```python
from build123d import *

# Parameters (mm, degrees)
SKETCH_2_R                   = 22.5
EXTRUDE_2_DEPTH              = 2
SKETCH_22_R                  = 10
CUT_EXTRUDE_1_DEPTH          = 2
FILLET_4_R                   = 0.2
SKETCH_54_R                  = 22.5
EXTRUDE_6_DEPTH              = 11
SKETCH_55_R                  = 18.5
CUT_EXTRUDE_2_DEPTH          = 8
HOLE_WIZARD_M4_1_D           = 4.5
HOLE_WIZARD_M4_1_CBORE_D     = 8
HOLE_WIZARD_M4_1_CBORE_DEPTH = 1
PATTERN_CIRCULAR_1_COUNT     = 3
SKETCH_59_R                  = 18.5
SKETCH_59_R_2                = 17.5
EXTRUDE_7_DEPTH              = 1
EXTRUDE_8_DEPTH              = 9
FILLET_6_R                   = 0.3
SKETCH_68_R                  = 9.5
CUT_EXTRUDE_7_DEPTH          = 7
SKETCH_69_R                  = 8.5
CUT_EXTRUDE_8_DEPTH          = 3
FILLET_7_R                   = 0.3


with BuildPart() as part:
    # 스케치2 → 보스-돌출2 (new body)
    with BuildSketch(Plane(origin=(0, 6, 0), x_dir=(1, 0, 0), z_dir=(0, 0, -1))):
        with Locations((0, 6)):
            Circle(SKETCH_2_R)
    extrude(amount=EXTRUDE_2_DEPTH)

    # 스케치22 → 컷-돌출1 (cut)
    with BuildSketch(Plane.XY):
        Circle(SKETCH_22_R)
    extrude(amount=-CUT_EXTRUDE_1_DEPTH, mode=Mode.SUBTRACT)

    # 필렛4
    fillet_4_edges = [part.edges().sort_by_distance(p)[0] for p in [
        (-10, 0, 0),
    ]]
    fillet(fillet_4_edges, radius=FILLET_4_R)

    # 스케치54 → 보스-돌출6 (add)
    with BuildSketch(Plane(origin=(0, 0, -2), x_dir=(-1, 0, 0), z_dir=(0, 0, -1))):
        Circle(SKETCH_54_R)
    extrude(amount=EXTRUDE_6_DEPTH)

    # 스케치55 → 컷-돌출2 (cut)
    with BuildSketch(Plane(origin=(0, 0, -13), x_dir=(-1, 0, 0), z_dir=(0, 0, -1))):
        Circle(SKETCH_55_R)
    extrude(amount=-CUT_EXTRUDE_2_DEPTH, mode=Mode.SUBTRACT)

    # M4 육각 소켓 머리 캡 나사용 카운터보어1 (through all)
    with Locations(Plane(origin=(0, 0, -5), x_dir=(-1, 0, 0), z_dir=(0, 0, -1))):
        with Locations((0, 6)):
            hole_wizard_m4_1 = CounterBoreHole(HOLE_WIZARD_M4_1_D / 2, HOLE_WIZARD_M4_1_CBORE_D / 2, HOLE_WIZARD_M4_1_CBORE_DEPTH)

    # 원형 패턴1: M4 육각 소켓 머리 캡 나사용 카운터보어1 ×3 about axis
    pattern_circular_1_axis = Axis((0, 0, 0), (0, 0, 1))
    for i in range(1, PATTERN_CIRCULAR_1_COUNT):
        add(hole_wizard_m4_1.rotate(pattern_circular_1_axis, i * 360 / PATTERN_CIRCULAR_1_COUNT), mode=Mode.SUBTRACT)

    # 스케치59 → 보스-돌출7 (add)
    with BuildSketch(Plane(origin=(0, 0, -5), x_dir=(-1, 0, 0), z_dir=(0, 0, -1))):
        Circle(SKETCH_59_R)
        Circle(SKETCH_59_R_2, mode=Mode.SUBTRACT)
    extrude(amount=EXTRUDE_7_DEPTH)

    # 스케치60 → 보스-돌출8 (add)
    with BuildSketch(Plane(origin=(0, 0, -13), x_dir=(-1, 0, 0), z_dir=(0, 0, -1))):
        with BuildLine():
            Line((-22.323526687, -2.8125), (-14.882351125, -61.875))
            ThreePointArc((-14.882351125, -61.875), (0, -75), (14.882351125, -61.875))
            Line((14.882351125, -61.875), (22.323526687, -2.8125))
            ThreePointArc((22.323526687, -2.8125), (0, -22.5), (-22.323526687, -2.8125))
        make_face()
    extrude(amount=-EXTRUDE_8_DEPTH)

    # 필렛6
    fillet_6_edges = [part.edges().sort_by_distance(p)[0] for p in [
        (18.5, 0, -6),
    ]]
    fillet(fillet_6_edges, radius=FILLET_6_R)

    # 스케치68 → 컷-돌출7 (cut)
    with BuildSketch(Plane.XY.offset(-4)):
        with Locations((0, -60)):
            Circle(SKETCH_68_R)
    extrude(amount=-CUT_EXTRUDE_7_DEPTH, mode=Mode.SUBTRACT)

    # 스케치69 → 컷-돌출8 (cut, through all)
    with BuildSketch(Plane.XY.offset(-11)):
        with Locations((0, -60)):
            Circle(SKETCH_69_R)
    extrude(amount=-CUT_EXTRUDE_8_DEPTH, mode=Mode.SUBTRACT)

    # 필렛7
    fillet_7_edges = [part.edges().sort_by_distance(p)[0] for p in [
        (-9.5, -60, -11),
    ]]
    fillet(fillet_7_edges, radius=FILLET_7_R)


solid = part.part
```
Here's how the part is built. I have some questions about the finished solid (model axes, mm). A direction names the side the tool comes from. Give positions to 0.01 mm unless a question says otherwise; leave off trailing zeros. Write each loop counter-clockwise with the first axis right and the second up, starting at its lowest first coordinate (ties: lowest second). Pieces come first, ordered by that corner, then holes. Notation, with made-up numbers: (74.25, -21.5) -> (92.25, -21.5) arc R18 cw to (92.25, 13.5) -> close; hole circle Ø10 at (13, 2.5). An arc over 180 degrees is marked (long way). Write each question's results on one line, items separated by ' | '.
Item 1: We'd pull the mould along Y, two halves only. Please class faces 1 (the face through (-3.118, -3.862, -2.986)), 2 (the face through (0, -38, -4)), 3 (the face through (-18.55, -32.76, -8.56)): pulls with the +Y half, pulls with the -Y half, needs draft (parallel to the pull), parting line crosses it, or undercut.
Output:
face 1: undercut | face 2: needs draft | face 3: pulls with the -Y half
Item 2: For pin 1 Ø7 at (x, y) = (5.2, -3) entering from -Z; pin 2 Ø2 at (x, y) = (-13.5, -2) entering from -Z; pin 3 Ø1 at (x, z) = (17, -9) entering from +Y, each with a flat end and sliding along its axis, tell me the tip position at first contact or that it passes through.
Output:
pin 1: stops at z = -4 | pin 2: stops at z = -5 | pin 3: stops at y = 15.3
Item 3: On a 3-axis mill with a long thin cutter (end or side, diameter ignored), from which of +Z, -Z, +X, -X, +Y, -Y can I reach the whole of each face in a straight line? I mean faces 4 (the face through (0, 0, -2)), 5 (the face through (18.655, -31.93, -8.563)), 6 (the face through (15, 10, -6)). Say none if no direction works.
Output:
face 4: +Z | face 5: +Z, -Z, +X, -Y | face 6: -Z
Item 4: Suppose I cut it at C-C on x = 0. Give the number of separate pieces and of enclosed holes in the cut face, plus the area to 3 significant figures.
Output:
separate pieces: 3 | enclosed holes: 0 | area: 540 mm^2
Item 5: If I drill on L1, parallel to Y at x = -2, z = -10; L2, parallel to Y at x = 0, z = -1.3; L3, parallel to Y at x = 7, z = -10.25, over which ranges is the centre line in solid material (lowest first)?
Output:
L1: y = -74.87 to -69.29, -50.71 to -18.39, 18.39 to 22.41 | L2: y = -22.5 to -10, 10 to 22.5 | L3: y = -73.27 to -66.42, -53.58 to -17.12, 17.12 to 21.38
Item 6: Suppose I cut it at A-A on z = -8.5. Write out the boundary of the cut face in (x, y) (1 decimal), plus the area to 3 significant figures.
Output:
outline: (-22.3, -2.8) -> (-14.9, -61.9) arc R15 ccw to (14.9, -61.9) -> (22.3, -2.8) arc R22.5 ccw (long way) to start; hole circle Ø37 at (0, 0); hole circle Ø19 at (0, -60) | area: 2,060 mm^2
Item 7: Suppose I cut it at D-D on y = -45.5. Write out the boundary of the cut face in (x, z).
Output:
outline: (-16.95, -13) -> (16.95, -13) -> (16.95, -4) -> (-16.95, -4) -> close
Item 8: Suppose I cut it at B-B on y = -60. Write out the boundary of the cut face in (x, z), plus the area to 3 significant figures.
Output:
outline: (-15.12, -13) -> (-8.5, -13) -> (-8.5, -11) -> (-9.2, -11) arc R0.3 cw to (-9.5, -10.7) -> (-9.5, -4) -> (-15.12, -4) -> close; (8.5, -13) -> (15.12, -13) -> (15.12, -4) -> (9.5, -4) -> (9.5, -10.7) arc R0.3 cw to (9.2, -11) -> (8.5, -11) -> close | area: 105 mm^2
